Model file for the job. Use its own axes, mm. A direction names the side the tool comes from. Give positions to 0.01 mm unless a question says otherwise; leave off trailing zeros. Order: outer loops, then holes, each group sorted by start corner. A loop starts at its lowest first (then second) coordinate and runs counter-clockwise, first axis right, second up. Notation, with made-up numbers: M -2.75,48 L 10.25,48 A30 cw 10.25,74 Z; hole C -31.75,21.25 d11. An arc over 180 degrees is marked long. Return JSON: item names as keys, results as strings. Group by question number.
1. Pin check, flat tips, straight feed: pin 1 (1 mm diameter, centred on x = -4.5, z = 16, fed in from -Y); pin 2 (2 mm diameter, centred on y = 3.5, z = 18, fed in from +X); pin 3 (2 mm diameter, centred on x = 1.5, y = 4, fed in from -Z); pin 4 (2 mm diameter, centred on y = 3, z = 19, fed in from -X). Stop position of each tip, or through.
2. 3-axis set-ups, long thin cutter, end or side, ignore diameter. For faces 1 (the face through (-2, 3, 15)), 2 (the face through (-0.1, -3.2, 0)): which of +Z, -Z, +X, -X, +Y, -Y reach the whole face in a straight line?
3. Wall check: probe 1 along Y at (x, z) = (0, 7); probe 2 along X at (y, z) = (-0.75, 2); probe 3 along X at (y, z) = (-0.25, 27). Give the ranges that are in metal, low to high. Write a range as [from, to].
4. Two-plate mould, pull along X, no slides. Class faces 3 (the face through (0, 4.236, 15)), 4 (the face through (-0.1, -3.2, 30)), 5 (the face through (-7.493, 0.33, 14.79)): released by +X, released by -X, zero draft, split by the parting line, or undercut.
5. Slice it at A-A on x = 0. List the corners of the cut face in (y, z), then the cut area to 3 significant figures.
6. Slice it at C-C on z = 27.75. List the corners of the cut face in (x, y), then the cut area to 3 significant figures.
7. Slice it at D-D on x = 3.5. List the corners of the cut face in (y, z).
8. Slice it at B-B on y = 0. List the corners of the cut face in (x, z), then the cut area to 3 significant figures.
from build123d import *

# Parameters (mm, degrees)
SKETCH1_R           = 7.5
SKETCH1_R_2         = 3
BOSS_EXTRUDE1_DEPTH = 30
CUT_EXTRUDE1_DEPTH  = 32.819805153


with BuildPart() as part:
    # Sketch1 → Boss-Extrude1 (new body)
    with BuildSketch(Plane.XY):
        Circle(SKETCH1_R)
        Circle(SKETCH1_R_2, mode=Mode.SUBTRACT)
    extrude(amount=BOSS_EXTRUDE1_DEPTH)

    # Sketch2 → Cut-Extrude1 (cut, through all)
    with BuildSketch(Plane.XY.offset(30)):
        with BuildLine():
            ThreePointArc((-2, 2.236067977), (-1.070466269, 2.802517077), (0, 3))
            Line((0, 3), (0, 4.236067977))
            Line((0, 4.236067977), (-2, 4.236067977))
            Line((-2, 4.236067977), (-2, 2.236067977))
        make_face()
        with BuildLine():
            Line((0, 4.236067977), (0, 3))
            ThreePointArc((0, 3), (1.070466269, 2.802517077), (2, 2.236067977))
            Line((2, 2.236067977), (2, 4.236067977))
            Line((2, 4.236067977), (0, 4.236067977))
        make_face()
    extrude(amount=-CUT_EXTRUDE1_DEPTH, mode=Mode.SUBTRACT)


solid = part.part
Result:
{
 "1": {"pin 1": "stops at y = -6.34", "pin 2": "stops at x = 7.07", "pin 3": "stops at z = 0", "pin 4": "stops at x = -7.23"},
 "2": {"face 1": "+Z, -Z", "face 2": "-Z, +X, -X, +Y, -Y"},
 "3": {"probe 1": "y = [-7.5, -3], [4.24, 7.5]", "probe 2": "x = [-7.46, -2.9], [2.9, 7.46]", "probe 3": "x = [-7.5, -2.99], [2.99, 7.5]"},
 "4": {"face 3": "undercut", "face 4": "zero draft", "face 5": "split by the parting line"},
 "5": {"outline": "M -7.5,0 L -3,0 L -3,30 L -7.5,30 Z; M 4.24,0 L 7.5,0 L 7.5,30 L 4.24,30 Z", "area": "233 mm2"},
 "6": {"outline": "C 0,0 d15; hole M -2,2.24 A3 ccw long 2,2.24 L 2,4.24 L -2,4.24 Z", "area": "143 mm2"},
 "7": {"outline": "M -6.63,0 L 6.63,0 L 6.63,30 L -6.63,30 Z"},
 "8": {"outline": "M -7.5,0 L -3,0 L -3,30 L -7.5,30 Z; M 3,0 L 7.5,0 L 7.5,30 L 3,30 Z", "area": "270 mm2"}
}
